from build123d import *

# Parameters (mm, degrees)
F0_R        = 13
F0_R_2      = 1.2126826201
F0_R_3      = 8
F0_R_4      = 7
F1_DEPTH    = 2
F2_DEPTH    = 6
F4_R        = 13
F4_R_2      = 8
F4_R_3      = 7
F5_DEPTH    = 1
F2_FACE_R   = 13
F2_FACE_R_2 = 1.2126826201
F6_DEPTH    = 1
F7_DEPTH    = 2
F8_R        = 4.999


# Not quite as in the source:
# - a fillet or chamfer is up to 0.001 mm smaller than in the source, because OpenCascade refuses the exact size


with BuildPart() as f1:
    # F0 (on Top) → F1 (new body)
    with BuildSketch(Plane.XY):
        Circle(F0_R)
        with Locations((0, -10.5861881748)):
            Circle(F0_R_2, mode=Mode.SUBTRACT)
        Circle(F0_R_3, mode=Mode.SUBTRACT)
        Circle(F0_R_3)
        Circle(F0_R_4, mode=Mode.SUBTRACT)
        Circle(F0_R_4)
    extrude(amount=F1_DEPTH)

    # F0 (on Top) → F2 (join)
    with BuildSketch(Plane.XY):
        Circle(F0_R)
        with Locations((0, -10.5861881748)):
            Circle(F0_R_2, mode=Mode.SUBTRACT)
        Circle(F0_R_3, mode=Mode.SUBTRACT)
    extrude(amount=F2_DEPTH)

    # F4 (on offset) → F5 (join)
    with BuildSketch(Plane.XY.offset(6)):
        Circle(F4_R)
        Circle(F4_R_2, mode=Mode.SUBTRACT)
        Circle(F4_R_2)
        Circle(F4_R_3, mode=Mode.SUBTRACT)
    extrude(amount=-F5_DEPTH)

    # F2_face (on face) + F0 (on Top) → F6 (join)
    with BuildSketch(Plane(origin=(0, 0.0929272063, 0), x_dir=(1, 0, 0), z_dir=(0, 0, -1))):
        with Locations((0, 0.0929272063)):
            Circle(F2_FACE_R)
        with Locations((0, 10.6791153811)):
            Circle(F2_FACE_R_2, mode=Mode.SUBTRACT)
    with BuildSketch(Plane.XY):
        Circle(F0_R_4)
    extrude(amount=-F6_DEPTH, dir=(0, 0, -1))

    # F0 (on Top) → F7 (join)
    with BuildSketch(Plane.XY):
        Circle(F0_R)
        with Locations((0, -10.5861881748)):
            Circle(F0_R_2, mode=Mode.SUBTRACT)
        Circle(F0_R_3, mode=Mode.SUBTRACT)
    extrude(amount=-F7_DEPTH)

    # F8 (radius 5 in the source; OpenCascade refuses exactly that, so slightly less here)
    f8_edges = [f1.edges().sort_by_distance(p)[0] for p in [
        (-13, 0, -2),
    ]]
    fillet(f8_edges, radius=F8_R)


solid = f1.part
Source: CAD feature listing. Evaluate the final solid. Frame: model axes, mm. A direction names the side the tool comes from. Coordinates: 2 decimals unless noted, no trailing zeros. Loops run counter-clockwise (first coordinate to the right, second up) from the corner with the lowest first, then second, coordinate; pieces in that order, holes last. Notation, with made-up numbers: (5.5, 72.5) - (21.5, 72.5) arc R22 cw to (21.5, 111.5) - close; hole circle Ø7 at (83, 40). An arc over 180 degrees is marked (long way). One line per item, written item: value. Start each with the question number.
1. Mould query, pull axis X, two halves, no side actions, for faces 4 (the cylindrical face through (-2.82, -12.69, 4.48)), 5 (the flat face through (6, -6, 6)), 6 (the flat face through (0, 0, 0)), 7 (the flat face through (4, -6, 5)). Classes: pulls with the +X half, pulls with the -X half, needs draft (parallel to the pull), parting line crosses it, or undercut.
2. Section A-A (z = 3.75). Return the cut outline in (x, y).
3. Contact query for flat-ended pins moving along their axis: P1, Ø1.5, axis at x = 8, z = 4.5, coming from the +Y side; P2, Ø2, axis at y = -9.5, z = -0.5, coming from the -X side; P3, Ø8.5, axis at x = 0, y = 0, coming from the +Z side. Output: stop coordinate, or through.
4. Set-up query: faces 1 (the cylindrical face through (-1.73, -7.81, -0.99)), 2 (the cylindrical face through (-1.73, -7.81, 3.48)), 3 (the cylindrical face through (6.466, -2.681, 5.507)). Return all of +Z, -Z, +X, -X, +Y, -Y with unobstructed straight access to the full face (end or side cutting, diameter ignored); none if empty.
5. Ray query, L1, parallel to Y at x = 0, z = 3.6; L2, parallel to Y at x = 0, z = 5.4; L3, parallel to Z at x = 2, y = -6.75. Return the intervals inside material, ascending.
Verdict:
1. face 4: parting line crosses it
1. face 5: needs draft
1. face 6: undercut
1. face 7: undercut
2. outline: circle Ø26 at (0, 0); hole circle Ø16 at (0, 0)
3. P1: stops at y = 10.79
3. P2: stops at x = -8.38
3. P3: stops at z = 2
4. face 1: -Z
4. face 2: none
4. face 3: +Z
5. L1: y = -13 to -8, 8 to 13
5. L2: y = -13 to -7, 7 to 13
5. L3: z = 0 to 2, 5 to 6
